Drawing for the job (mm, zero at the part's lowest x, y, z). Give positions to 0.01 mm unless a question says otherwise; leave off trailing zeros. Loops run counter-clockwise (first coordinate to the right, second up) from the corner with the lowest first, then second, coordinate; pieces in that order, holes last. Notation, with made-up numbers: (22.25, 59.25) -> (62.25, 59.25) arc R36 cw to (62.25, 95.25) -> close; hole circle Ø1 at (-5, 3.5). An arc over 180 degrees is marked (long way). Use CSV: the item, a comma, the result in double quotes. Start each with the question number.
(1) Cut at B-B on z = 889. Write the cut outline in (x, y).
(2) Flat gauge pins, fed straight in: pin 1 (8 mm diameter, centred on x = 1071, y = 103.5, fed in from +Z); pin 2 (6 mm diameter, centred on y = 213.5, z = 658, fed in from +X); pin 3 (8 mm diameter, centred on x = 690.5, y = 354, fed in from -Z); pin 4 (12 mm diameter, centred on x = 938.5, y = 114, fed in from +Z) (1 decimal). Where does each tip first touch, or does it go through?
(3) Cut at A-A on x = 1270. Write the cut outline in (y, z), then the cut area to 3 significant figures.
(4) Cut at D-D on y = 122. Write the cut outline in (x, z).
(5) Cut at C-C on y = 229.5. Write the cut outline in (x, z), then the cut area to 3 significant figures.
(6) Drill centre lines: probe 1 along Z at (x, y) = (741.5, 63); probe 2 along Z at (x, y) = (1270, 28); probe 3 along X at (y, z) = (6.75, 838.2). Where is each one in solid material? Low to high.
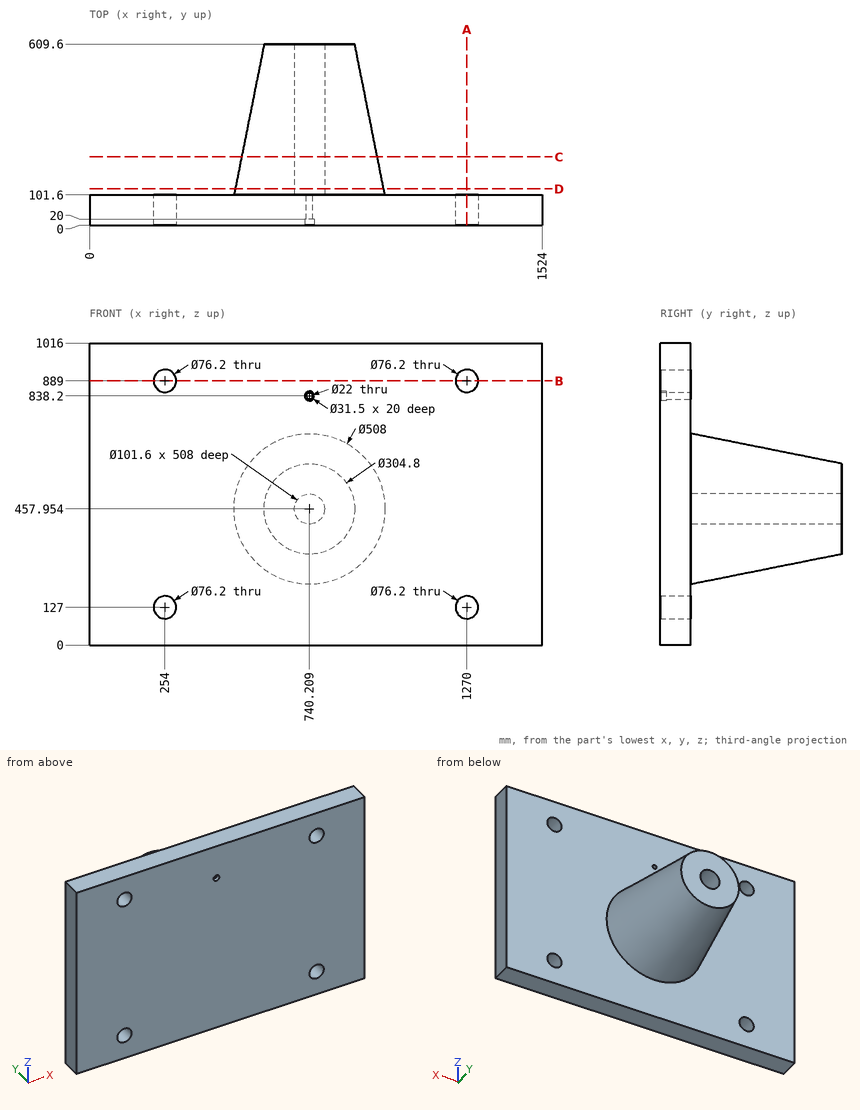
Check result:
1,outline,"(0, 0) -> (215.9, 0) -> (215.9, 101.6) -> (0, 101.6) -> close; (292.1, 0) -> (1231.9, 0) -> (1231.9, 101.6) -> (292.1, 101.6) -> close; (1308.1, 0) -> (1524, 0) -> (1524, 101.6) -> (1308.1, 101.6) -> close"
2,pin 1,"z = 1016"
2,pin 2,"x = 862.08"
2,pin 3,"z = 259.32"
2,pin 4,"z = 620.3"
3,outline,"(0, 0) -> (101.6, 0) -> (101.6, 88.9) -> (0, 88.9) -> close; (0, 165.1) -> (101.6, 165.1) -> (101.6, 850.9) -> (0, 850.9) -> close; (0, 927.1) -> (101.6, 927.1) -> (101.6, 1016) -> (0, 1016) -> close"
3,area,"87,700 mm²"
4,outline,"circle Ø499.84 at (740.21, 457.95); hole circle Ø101.6 at (740.21, 457.95)"
5,outline,"circle Ø456.84 at (740.21, 457.95); hole circle Ø101.6 at (740.21, 457.95)"
5,area,"156,000 mm²"
6,probe 1,"0 to 827.28, 849.12 to 1016"
6,probe 2,"0 to 88.9, 165.1 to 850.9, 927.1 to 1016"
6,probe 3,"0 to 724.46, 755.96 to 1524"
